from build123d import *

# Parameters (mm, degrees)
SKETCH6_R                = 56
BOSS_EXTRUDE3_DEPTH      = 5
CUT_EXTRUDE4_DEPTH       = 1
CUT_EXTRUDE4_DEPTH_BACK  = 6
SKETCH7_8_R              = 2
CUT_EXTRUDE5_DEPTH       = 1
CUT_EXTRUDE5_DEPTH_BACK  = 6
SKETCH10_R               = 2
SKETCH11_R               = 2.5
CUT_EXTRUDE14_DEPTH      = 6
CUT_EXTRUDE14_DEPTH_BACK = 5
SKETCH12_R               = 9
BOSS_EXTRUDE4_DEPTH      = 4


with BuildPart() as part:
    # Sketch6 → Boss-Extrude3 (new body)
    with BuildSketch(Plane(origin=(0, 0, 0), x_dir=(1, 0, 0), z_dir=(0, 1, 0))):
        Circle(SKETCH6_R)
    extrude(amount=BOSS_EXTRUDE3_DEPTH)

    # Sketch7 → Cut-Extrude4 (cut, two sides)
    with BuildSketch(Plane(origin=(0, 5, 0), x_dir=(1, 0, 0), z_dir=(0, 1, 0))) as cut_extrude4_sk:
        with BuildLine():
            Line((20.503283661, 14.304382514), (36.669318151, 25.582826732))
            ThreePointArc((36.669318151, 25.582826732), (31.677302024, 31.554214517), (25.725394502, 36.569440726))
            Line((25.725394502, 36.569440726), (14.384097861, 20.447438195))
            ThreePointArc((14.384097861, 20.447438195), (17.712047613, 17.64322446), (20.503283661, 14.304382514))
        make_face()
        with BuildLine():
            Line((4.631236844, 24.567288114), (8.282785337, 43.937630618))
            ThreePointArc((8.282785337, 43.937630618), (0, 44.711518844), (-8.282785337, 43.937630618))
            Line((-8.282785337, 43.937630618), (-4.631236844, 24.567288114))
            ThreePointArc((-4.631236844, 24.567288114), (0, 25), (4.631236844, 24.567288114))
        make_face()
        with BuildLine():
            Line((-14.304382514, 20.503283661), (-25.582826732, 36.669318151))
            ThreePointArc((-25.582826732, 36.669318151), (-31.554214517, 31.677302024), (-36.569440726, 25.725394502))
            Line((-36.569440726, 25.725394502), (-20.447438195, 14.384097861))
            ThreePointArc((-20.447438195, 14.384097861), (-17.64322446, 17.712047613), (-14.304382514, 20.503283661))
        make_face()
        with BuildLine():
            Line((-24.567288114, 4.631236844), (-43.937630618, 8.282785337))
            ThreePointArc((-43.937630618, 8.282785337), (-44.711518844, 0), (-43.937630618, -8.282785337))
            Line((-43.937630618, -8.282785337), (-24.567288114, -4.631236844))
            ThreePointArc((-24.567288114, -4.631236844), (-25, 0), (-24.567288114, 4.631236844))
        make_face()
        with BuildLine():
            ThreePointArc((-36.669318151, -25.582826732), (-31.677302024, -31.554214517), (-25.725394502, -36.569440726))
            Line((-25.725394502, -36.569440726), (-14.384097861, -20.447438195))
            ThreePointArc((-14.384097861, -20.447438195), (-17.712047613, -17.64322446), (-20.503283661, -14.304382514))
            Line((-20.503283661, -14.304382514), (-36.669318151, -25.582826732))
        make_face()
        with BuildLine():
            ThreePointArc((-8.282785337, -43.937630618), (0, -44.711518844), (8.282785337, -43.937630618))
            Line((8.282785337, -43.937630618), (4.631236844, -24.567288114))
            ThreePointArc((4.631236844, -24.567288114), (0, -25), (-4.631236844, -24.567288114))
            Line((-4.631236844, -24.567288114), (-8.282785337, -43.937630618))
        make_face()
        with BuildLine():
            ThreePointArc((25.582826732, -36.669318151), (31.554214517, -31.677302024), (36.569440726, -25.725394502))
            Line((36.569440726, -25.725394502), (20.447438195, -14.384097861))
            ThreePointArc((20.447438195, -14.384097861), (17.64322446, -17.712047613), (14.304382514, -20.503283661))
            Line((14.304382514, -20.503283661), (25.582826732, -36.669318151))
        make_face()
        with BuildLine():
            ThreePointArc((44.711518844, 0), (44.517626378, 4.159430127), (43.937630618, 8.282785337))
            Line((43.937630618, 8.282785337), (24.567288114, 4.631236844))
            ThreePointArc((24.567288114, 4.631236844), (24.891586961, 2.325703887), (25, 0))
            ThreePointArc((25, 0), (24.891586961, -2.325703887), (24.567288114, -4.631236844))
            Line((24.567288114, -4.631236844), (43.937630618, -8.282785337))
            ThreePointArc((43.937630618, -8.282785337), (44.517626378, -4.159430127), (44.711518844, 0))
        make_face()
    extrude(amount=CUT_EXTRUDE4_DEPTH, mode=Mode.SUBTRACT)
    extrude(cut_extrude4_sk.sketch, amount=-CUT_EXTRUDE4_DEPTH_BACK, mode=Mode.SUBTRACT)

    # Sketch7<8> → Cut-Extrude5 (cut, two sides)
    with BuildSketch(Plane(origin=(0, 5, 0), x_dir=(1, 0, 0), z_dir=(0, 1, 0))) as cut_extrude5_sk:
        with Locations((19.298680627, 8.282785337)):
            Circle(SKETCH7_8_R)
        with Locations((19.736681401, -7.225357928)):
            Circle(SKETCH7_8_R)
        with Locations((8.023054044, 18.938985285)):
            Circle(SKETCH7_8_R)
        with Locations((9.080481453, -18.500984511)):
            Circle(SKETCH7_8_R)
        with Locations((-7.485089221, 18.500984511)):
            Circle(SKETCH7_8_R)
        with Locations((-6.427661812, -18.938985285)):
            Circle(SKETCH7_8_R)
        with Locations((-18.141289169, 7.225357928)):
            Circle(SKETCH7_8_R)
        with Locations((-17.703288395, -8.282785337)):
            Circle(SKETCH7_8_R)
    extrude(amount=CUT_EXTRUDE5_DEPTH, mode=Mode.SUBTRACT)
    extrude(cut_extrude5_sk.sketch, amount=-CUT_EXTRUDE5_DEPTH_BACK, mode=Mode.SUBTRACT)

    # Sketch10 → Cut-Revolve1 (revolve, cut)
    with BuildSketch(Plane.XY):
        with Locations((56, 2.5)):
            Circle(SKETCH10_R)
    revolve(axis=Axis((0, 40.614262211, 0), (0, -1, 0)), mode=Mode.SUBTRACT)

    # Sketch11 → Cut-Extrude14 (cut, two sides)
    with BuildSketch(Plane(origin=(0, 0, 0), x_dir=(1, 0, 0), z_dir=(0, 1, 0))) as cut_extrude14_sk:
        Circle(SKETCH11_R)
    extrude(amount=CUT_EXTRUDE14_DEPTH, mode=Mode.SUBTRACT)
    extrude(cut_extrude14_sk.sketch, amount=-CUT_EXTRUDE14_DEPTH_BACK, mode=Mode.SUBTRACT)

    # Sketch12 → Boss-Extrude4 (add)
    with BuildSketch(Plane(origin=(0, 0, 0), x_dir=(1, 0, 0), z_dir=(0, 1, 0))):
        Circle(SKETCH12_R)
        Polygon((0, 7), (-6.062177826, 3.5), (-6.062177826, -3.5), (0, -7), (6.062177826, -3.5), (6.062177826, 3.5), align=None, mode=Mode.SUBTRACT)
    extrude(amount=-BOSS_EXTRUDE4_DEPTH)


solid = part.part
Verification items for the finished model (mm, model axes). A direction names the side the tool comes from. Coordinates: 2 decimals unless noted, no trailing zeros.
1. Set-up check for faces 5 (the face through (-20.134, 2.535, 28.621)), 6 (the face through (-2.1, -4, -6.1)), 7 (the face through (-3.074, -1.972, 5.226)): record each of +Z, -Z, +X, -X, +Y, -Y from which the full face is reachable in a straight line by a thin tool's end or side.
Results found:
face 5: +Y, -Y
face 6: +Z, -Z, +X, -X, -Y
face 7: -Y
2. Release check for a two-part mould opening along X. For faces 1 (the face through (-1, 5, 12)), 2 (the face through (6.062, -2, 0)), 3 (the face through (-28.473, 2.535, 19.865)), 4 (the face through (51.73, 0.25, 21.45)) record: +X half, -X half, draft (parallel to the pull), parting line (faces both ways), or undercut.
Results found:
face 1: draft
face 2: undercut
face 3: undercut
face 4: parting line
3. Scan lines: line 1 (Z direction, x = -4, y = 3.75); line 2 (Z direction, x = 27.5, y = 4); line 3 (Z direction, x = -36, y = 2.5). Record each from-to range of solid material in increasing order.
Results found:
line 1: z = -54.29 to -44.53, -24.68 to 24.68, 44.53 to 54.29
line 2: z = -47.26 to -35.25, -19.19 to -5.18, 5.18 to 19.35, 35.25 to 47.26
line 3: z = -40.25 to -26.52, -25.32 to -6.79, 6.79 to 25.12, 26.52 to 40.25
4. Sectioned sample at A-A, the plane z = 22.5. Give the number of separate pieces and of enclosed holes in the cut face, and give its area (3 significant figures).
Results found:
separate pieces: 3
enclosed holes: 0
area: 335 mm2
5. Go/stop test with flat-tipped pins: pin 1 Ø5 at (x, z) = (-17.7, 8.28) entering from -Y; pin 2 Ø5 at (y, z) = (2, 36) entering from -X; pin 3 Ø1.2 at (y, z) = (-1.5, 0.5) entering from +X. Record where each tip stops, or that it passes through.
Results found:
pin 1: stops at y = 0
pin 2: stops at x = -44.5
pin 3: stops at x = 9
